Part model, mm, in its own coordinate system. A direction names the side the tool comes from. Coordinates: 2 decimals unless noted, no trailing zeros. Loops run counter-clockwise (first coordinate to the right, second up) from the corner with the lowest first, then second, coordinate; pieces in that order, holes last. Notation, with made-up numbers: (-36, 72) -> (18, 72) arc R18 cw to (18, 85) -> close; hole circle Ø10 at (51, 74). An arc over 180 degrees is marked (long way). One line per question, with ' | ' between items. Start each with the question number.
1) Drop flat-ended pins along their axis: pin 1 (2.5 mm diameter, centred on x = -8.6, z = -11, fed in from +Y); pin 2 (3.5 mm diameter, centred on x = 8.6, z = 11, fed in from -Y); pin 3 (3 mm diameter, centred on x = 11, y = -17.5, fed in from -Z); pin 4 (2.5 mm diameter, centred on x = 19.5, y = -13, fed in from +Z). Give the stop position or say it passes through.
2) Cut at C-C (z = -33.5). List the corners of the cut face in (x, y), plus the area to 3 significant figures.
3) Two-plate mould, pull along X, no slides. Class faces 4 (the face through (12, -12, -24)), 5 (the face through (19.7, -11.9, -11.5)), 6 (the face through (0, -13, 8)): released by +X, released by -X, zero draft, split by the parting line, or undercut.
4) 3-axis set-ups, long thin cutter, end or side, ignore diameter. For faces 1 (the face through (10.798, -2.958, 11.097)), 2 (the face through (0, -13, 14)), 3 (the face through (19.7, -11.9, 18.5)): which of +Z, -Z, +X, -X, +Y, -Y reach the whole face in a straight line?
5) Cut at A-A (x = 18.5). List the corners of the cut face in (y, z), plus the area to 3 significant figures.
6) Probe L1, parallel to Z at x = 0, y = -18.75; L2, parallel to Z at x = 9, y = -18.25; L3, parallel to Z at x = -0.5, y = -14.25. List the from-to ranges inside material, lowest first. Write a range as from..to.
7) Cut at B-B (x = 0). Count the separate pieces of the cut face and the enclosed holes in it, plus the area to 3 significant figures.
from build123d import *

# Parameters (mm, degrees)
F0_R         = 6
F0_W         = 15
F0_H         = 30
F1_DEPTH     = 25
F2_R         = 8.1
F2_R_2       = 6
F3_DEPTH     = 10
F4_R         = 8.1
F4_R_2       = 6
F5_DEPTH     = 10
F6_R         = 4
F7_DEPTH     = 39.001
F8_R         = 10
F9_T1_DEPTH  = 5
F9_T6_ANGLE  = 161.6623328293
F9_T11_ANGLE = 161.6623328293
F9_T16_ANGLE = 161.6623328293
F9_T21_ANGLE = 161.6623328293
F10_R        = 2.2
F11_DEPTH    = 11.6603414823
F12_R        = 2.2
F13_DEPTH    = 11.6603414823
F14_R        = 1.6
F14_W        = 10
F14_H        = 6
F15_DEPTH    = 25.0010004328
F16_R        = 2.2
F16_R_2      = 1.6
F17_DEPTH    = 6
F18_R        = 2.2
F19_DEPTH    = 6


# Not quite as in the source:
# - a fillet or chamfer that OpenCascade refuses, or shapes differently, is made with other operations: its cross-section is extruded or revolved along the edge and cut away or added


with BuildPart() as f1:
    # F0 (on Front) → F1 (new body)
    with BuildSketch(Plane.XZ):
        with BuildLine():
            Line((12, 18.5), (12, 35.5))
            ThreePointArc((12, 35.5), (0, 23.5), (-12, 35.5))
            Line((-12, 35.5), (-12, -35.5))
            ThreePointArc((-12, -35.5), (0, -23.5), (12, -35.5))
            Line((12, -35.5), (12, -11.5))
            Line((12, -11.5), (12, 18.5))
        make_face()
        with BuildLine():
            ThreePointArc((-12, 35.5), (0, 23.5), (12, 35.5))
            ThreePointArc((12, 35.5), (0, 47.5), (-12, 35.5))
        make_face()
        with Locations((0, 35.5)):
            Circle(F0_R, mode=Mode.SUBTRACT)
        with BuildLine():
            ThreePointArc((12, -35.5), (0, -23.5), (-12, -35.5))
            ThreePointArc((-12, -35.5), (0, -47.5), (12, -35.5))
        make_face()
        with Locations((0, -35.5)):
            Circle(F0_R, mode=Mode.SUBTRACT)
        with Locations((19.5, 3.5)):
            Rectangle(F0_W, F0_H)
    extrude(amount=F1_DEPTH)

    # F2 (on face) → F3 (cut)
    with BuildSketch(Plane.XZ.offset(25)):
        with Locations((0, 35.5)):
            Circle(F2_R)
        with Locations((0, 35.5)):
            Circle(F2_R_2, mode=Mode.SUBTRACT)
        with Locations((0, -35.5)):
            Circle(F2_R)
        with Locations((0, -35.5)):
            Circle(F2_R_2, mode=Mode.SUBTRACT)
    extrude(amount=-F3_DEPTH, mode=Mode.SUBTRACT)

    # F4 (on face) → F5 (cut)
    with BuildSketch(Plane(origin=(0, 0, 0), x_dir=(-1, 0, 0), z_dir=(0, 1, 0))):
        with Locations((0, 35.5)):
            Circle(F4_R)
        with Locations((0, 35.5)):
            Circle(F4_R_2, mode=Mode.SUBTRACT)
        with Locations((0, -35.5)):
            Circle(F4_R)
        with Locations((0, -35.5)):
            Circle(F4_R_2, mode=Mode.SUBTRACT)
    extrude(amount=-F5_DEPTH, mode=Mode.SUBTRACT)

    # F6 (on face) → F7 (cut, through all)
    with BuildSketch(Plane.YZ.offset(27)):
        with Locations((-12.5, 3.5)):
            Circle(F6_R)
    extrude(amount=-F7_DEPTH, mode=Mode.SUBTRACT)

    # F8
    f8_edges = [f1.edges().sort_by_distance(p)[0] for p in [
        (19.5, -25, 18.5),
        (19.5, 0, 18.5),
        (19.5, -25, -11.5),
        (19.5, 0, -11.5),
    ]]
    fillet(f8_edges, radius=F8_R)

    # F9: fillet of radius 5 on 6 edges, made by hand

    # F9_s2 → F9_t1 (join)
    with BuildSketch(Plane.XZ.offset(10)):
        with BuildLine():
            ThreePointArc((11.9996, 23.5009656854), (13.4644660941, 19.9644660941), (17.0009656854, 18.4996))
            Line((17.0009656854, 18.4996), (17.0009656854, 17.9994634315))
            ThreePointArc((17.0009656854, 17.9994634315), (14.5004828427, 17.9998634315), (12, 17.9998634315))
            Line((12, 17.9998634315), (11.4998634315, 18.5))
            ThreePointArc((11.4998634315, 18.5), (11.4998634315, 21.0004828427), (11.4994634315, 23.5009656854))
            Line((11.4994634315, 23.5009656854), (11.9996, 23.5009656854))
        make_face()
        with BuildLine():
            ThreePointArc((11.9996, -16.5009656854), (13.4644660941, -12.9644660941), (17.0009656854, -11.4996))
            Line((17.0009656854, -11.4996), (17.0009656854, -10.9994634315))
            ThreePointArc((17.0009656854, -10.9994634315), (14.5004828427, -10.9998634315), (12, -10.9998634315))
            Line((12, -10.9998634315), (11.4998634315, -11.5))
            ThreePointArc((11.4998634315, -11.5), (11.4998634315, -14.0004828427), (11.4994634315, -16.5009656854))
            Line((11.4994634315, -16.5009656854), (11.9996, -16.5009656854))
        make_face()
    extrude(amount=F9_T1_DEPTH)


with BuildPart() as f9_tool4:
    # F9_s5 → F9_t6 (revolve)
    with BuildSketch(Plane(origin=(0, -6.4717245278, -2.1450392426), x_dir=(1, 0, 0), z_dir=(0, -0.9492188488, -0.3146165557))):
        with BuildLine():
            ThreePointArc((11.9996, -3.7864399137), (13.4644660941, -0.2499403224), (17.0009656854, 1.2149257717))
            Line((17.0009656854, 1.2149257717), (17.0009656854, 1.7150623402))
            ThreePointArc((17.0009656854, 1.7150623402), (14.5004828427, 1.7146623402), (12, 1.7146623402))
            Line((12, 1.7146623402), (11.4998634315, 1.2145257717))
            ThreePointArc((11.4998634315, 1.2145257717), (11.4998634315, -1.285957071), (11.4994634315, -3.7864399137))
            Line((11.4994634315, -3.7864399137), (11.9996, -3.7864399137))
        make_face()
    revolve(axis=Axis((12, -10, 8.5), (1, 0, 0)), revolution_arc=F9_T6_ANGLE)

    split(bisect_by=Plane.XZ, keep=Keep.TOP)


with BuildPart() as f1_1:
    add(f1.part)

    # F9_t3: union F9_tool4
    add(f9_tool4.part)


with BuildPart() as f9_tool9:
    # F9_s10 → F9_t11 (revolve)
    with BuildSketch(Plane(origin=(0, -16.053686044, 5.3209598778), x_dir=(1, 0, 0), z_dir=(0, 0.9492188488, -0.3146165557))):
        with BuildLine():
            ThreePointArc((11.9996, 11.6518538065), (13.4644660941, 8.1153542151), (17.0009656854, 6.650488121))
            Line((17.0009656854, 6.650488121), (17.0009656854, 6.1503515525))
            ThreePointArc((17.0009656854, 6.1503515525), (14.5004828427, 6.1507515525), (12, 6.1507515525))
            Line((12, 6.1507515525), (11.4998634315, 6.650888121))
            ThreePointArc((11.4998634315, 6.650888121), (11.4998634315, 9.1513709638), (11.4994634315, 11.6518538065))
            Line((11.4994634315, 11.6518538065), (11.9996, 11.6518538065))
        make_face()
    revolve(axis=Axis((12, -15, 8.5), (-1, 0, 0)), revolution_arc=F9_T11_ANGLE)

    split(bisect_by=Plane.XZ.offset(25), keep=Keep.BOTTOM)


with BuildPart() as f1_2:
    add(f1_1.part)

    # F9_t8: union F9_tool9
    add(f9_tool9.part)


with BuildPart() as f9_tool14:
    # F9_s15 → F9_t16 (revolve)
    with BuildSketch(Plane(origin=(0, -8.5622042815, 2.8379242825), x_dir=(1, 0, 0), z_dir=(0, -0.9492188488, 0.3146165557))):
        with BuildLine():
            ThreePointArc((17.0009656854, 5.4296061697), (13.4644660941, 6.8944722638), (11.9996, 10.4309718552))
            Line((11.9996, 10.4309718552), (11.4994634315, 10.4309718552))
            ThreePointArc((11.4994634315, 10.4309718552), (11.4998634315, 7.9304890124), (11.4998634315, 5.4300061697))
            Line((11.4998634315, 5.4300061697), (12, 4.9298696012))
            ThreePointArc((12, 4.9298696012), (14.5004828427, 4.9298696012), (17.0009656854, 4.9294696012))
            Line((17.0009656854, 4.9294696012), (17.0009656854, 5.4296061697))
        make_face()
    revolve(axis=Axis((12, -10, -1.5), (-1, 0, 0)), revolution_arc=F9_T16_ANGLE)

    split(bisect_by=Plane.XZ, keep=Keep.TOP)


with BuildPart() as f1_3:
    add(f1_2.part)

    # F9_t13: union F9_tool14
    add(f9_tool14.part)


with BuildPart() as f9_tool19:
    # F9_s20 → F9_t21 (revolve)
    with BuildSketch(Plane(origin=(0, -13.9632062903, -4.6280748379), x_dir=(1, 0, 0), z_dir=(0, 0.9492188488, 0.3146165557))):
        with BuildLine():
            ThreePointArc((11.9996, -18.2963857479), (13.4644660941, -14.7598861565), (17.0009656854, -13.2950200625))
            Line((17.0009656854, -13.2950200625), (17.0009656854, -12.7948834939))
            ThreePointArc((17.0009656854, -12.7948834939), (14.5004828427, -12.7952834939), (12, -12.7952834939))
            Line((12, -12.7952834939), (11.4998634315, -13.2954200625))
            ThreePointArc((11.4998634315, -13.2954200625), (11.4998634315, -15.7959029052), (11.4994634315, -18.2963857479))
            Line((11.4994634315, -18.2963857479), (11.9996, -18.2963857479))
        make_face()
    revolve(axis=Axis((12, -15, -1.5), (1, 0, 0)), revolution_arc=F9_T21_ANGLE)

    split(bisect_by=Plane.XZ.offset(25), keep=Keep.BOTTOM)


with BuildPart() as f1_4:
    add(f1_3.part)

    # F9_t18: union F9_tool19
    add(f9_tool19.part)

    # F10 (on face) → F11 (cut, through all)
    with BuildSketch(Plane.XY.offset(18.5)):
        with Locations((22, -12.5)):
            Circle(F10_R)
    extrude(amount=-F11_DEPTH, mode=Mode.SUBTRACT)

    # F12 (on face) → F13 (cut, through all)
    with BuildSketch(Plane(origin=(0, 0, -11.5), x_dir=(1, 0, 0), z_dir=(0, 0, -1))):
        with Locations((22, 12.5)):
            Circle(F12_R)
    extrude(amount=-F13_DEPTH, mode=Mode.SUBTRACT)

    # F14 (on face) → F15 (cut, through all)
    with BuildSketch(Plane.XZ.offset(25)):
        with Locations((-8.6, 11)):
            Circle(F14_R)
        with Locations((0, 11)):
            Rectangle(F14_W, F14_H)
        with Locations((8.6, 11)):
            Circle(F14_R)
        with Locations((8.6, -11)):
            Circle(F14_R)
        with Locations((0, -11)):
            Rectangle(F14_W, F14_H)
        with Locations((-8.6, -11)):
            Circle(F14_R)
    extrude(amount=-F15_DEPTH, mode=Mode.SUBTRACT)

    # F16 (on face) → F17 (cut)
    with BuildSketch(Plane.XZ.offset(25)):
        with Locations((-8.6, 11)):
            Circle(F16_R)
        with Locations((-8.6, 11)):
            Circle(F16_R_2, mode=Mode.SUBTRACT)
        with Locations((8.6, 11)):
            Circle(F16_R)
        with Locations((8.6, 11)):
            Circle(F16_R_2, mode=Mode.SUBTRACT)
        with Locations((8.6, -11)):
            Circle(F16_R)
        with Locations((8.6, -11)):
            Circle(F16_R_2, mode=Mode.SUBTRACT)
        with Locations((-8.6, -11)):
            Circle(F16_R)
        with Locations((-8.6, -11)):
            Circle(F16_R_2, mode=Mode.SUBTRACT)
    extrude(amount=-F17_DEPTH, mode=Mode.SUBTRACT)

    # F18 (on face) → F19 (cut)
    with BuildSketch(Plane(origin=(0, 0, 0), x_dir=(-1, 0, 0), z_dir=(0, 1, 0))):
        with Locations((8.6, 11)):
            Circle(F18_R)
        with Locations((-8.6, 11)):
            Circle(F18_R)
        with Locations((-8.6, -11)):
            Circle(F18_R)
        with Locations((8.6, -11)):
            Circle(F18_R)
    extrude(amount=-F19_DEPTH, mode=Mode.SUBTRACT)


solid = f1_4.part
Reported:
1) pin 1: passes through | pin 2: stops at y = -19 | pin 3: stops at z = -42.83 | pin 4: stops at z = 18.5
2) outline: (-12, -25) -> (-7.85, -25) -> (-7.85, -15) -> (-5.66, -15) -> (-5.66, -10) -> (-7.85, -10) -> (-7.85, 0) -> (-12, 0) -> close; (5.66, -15) -> (7.85, -15) -> (7.85, -25) -> (12, -25) -> (12, 0) -> (7.85, 0) -> (7.85, -10) -> (5.66, -10) -> close | area: 229 mm²
3) face 4: released by +X | face 5: zero draft | face 6: undercut
4) face 1: +Y | face 2: +Y, -Y | face 3: +Z, +X, +Y, -Y
5) outline: (-25, -1.5) arc R10 ccw to (-15, -11.5) -> (-10, -11.5) arc R10 ccw to (0, -1.5) -> (0, 8.5) arc R10 ccw to (-10, 18.5) -> (-15, 18.5) arc R10 ccw to (-25, 8.5) -> close; hole circle Ø8 at (-12.5, 3.5) | area: 614 mm²
6) L1: z = -47.5..-43.6, -27.4..-14, -8..8, 14..27.4, 43.6..47.5 | L2: z = -43.44..-12.55, -9.45..9.45, 12.55..43.44 | L3: z = -47.49..-41.48, -29.52..-14, -8..-0.1, 7.1..8, 14..29.52, 41.48..47.49
7) separate pieces: 5 | enclosed holes: 1 | area: 1,260 mm²
